Could you check a few things on this model? Use its own coordinates, in mm. A direction names the side the tool comes from. Round coordinates to 2 decimals unless told otherwise and drop trailing zeros. Write each loop counter-clockwise with the first axis right and the second up, starting at its lowest first coordinate (ties: lowest second). Pieces come first, ordered by that corner, then holes. Notation, with made-up numbers: M 23,-38 L 69,-38 A23 ccw 69,-19 Z; hole C 76.25,67 d9. An arc over 180 degrees is marked long. One line per item, written item: value. Start each with the question number.
(1) I'm going to push a flat-ended pin straight in: pin 1 Ø1 at (x, z) = (-28.5, 6.5) entering from +Y. Where does the tip first touch, or does it pass through?
(2) If I drill on L1, parallel to Z at x = 28, y = 0.5; L2, parallel to Z at x = 0, y = 3.05; L3, parallel to X at y = 0.4, z = -1.5, over which ranges is the centre line in solid material (lowest first)?
(3) I want a section at C-C on z = 0. Count the separate pieces of the cut face and the enclosed holes in it, and give its area (3 significant figures).
(4) Thinking about a two-plate mould opening in X: for faces 1 (the face through (49.638, 1.014, -0.189)), 2 (the face through (27, 2, -8.5)), 3 (the face through (-9, 2, 13.5)), which applies, released by +X, released by -X, zero draft, split by the parting line, or undercut?
(5) Which directions (+Z, -Z, +X, -X, +Y, -Y) give clear straight access to the entire face, cutting with the end or side of a thin tool? Please do faces 4 (the face through (1, 4, 6)), 5 (the face through (41.498, 1.972, -0.187)).
(6) I want a section at D-D on x = -30.5. Please give me the cut outline in (y, z).
(7) I want a section at B-B on y = 3.25. Please give me the cut outline in (x, z), and give its area (3 significant figures).
(8) I want a section at A-A on x = 0. Please give me the cut outline in (y, z), and give its area (3 significant figures).
Autodesk Inventor part; units mm, degrees
ref_plane "YZ Plane" through (0, 0, 0) normal (1, 0, 0) x (0, 1, 0)
ref_plane "XZ Plane" through (0, 0, 0) normal (0, 1, 0) x (-1, 0, 0)
ref_plane "XY Plane" through (0, 0, 0) normal (0, 0, 1) x (1, 0, 0)
sketch "Sketch1" plane through (0, 0, 0) normal (0, 1, 0) x (-1, 0, 0)
  circle A0 centre (0, 0) radius 13.5
  circle A1 centre (0, 0) radius 60
  line L0 (-58.4615, -13.5) -> (58.4615, -13.5)
  line L1 (58.4615, -13.5) -> (58.4615, 13.5)
  line L2 (58.4615, 13.5) -> (-58.4615, 13.5)
  line L3 (-58.4615, 13.5) -> (-58.4615, -13.5)
  line L4 (-58.4615, -13.5) -> (58.4615, 13.5) construction
  line L5 (58.4615, -13.5) -> (-58.4615, 13.5) construction
  line L6 (-20, 0) -> (-33, 0) construction
  line L7 (-20, 8.5) -> (-33, 8.5)
  line L8 (-33, -8.5) -> (-20, -8.5)
  arc A2 (-20, -8.5) -> (-20, 8.5) centre (-20, 0) ccw
  arc A3 (-33, 8.5) -> (-33, -8.5) centre (-33, 0) ccw
  line L9 (-58.4615, -13.5) -> (-42.8731, 13.5)
  line L10 (-58.4615, -13.5) -> (-27.2846, -13.5) construction
  line L11 (33, 0) -> (20, 0) construction
  line L12 (33, 8.5) -> (20, 8.5)
  line L13 (20, -8.5) -> (33, -8.5)
  arc A4 (33, -8.5) -> (33, 8.5) centre (33, 0) ccw
  arc A5 (20, 8.5) -> (20, -8.5) centre (20, 0) ccw
  line L14 (58.4615, 13.5) -> (47.2814, -5.8645)
  line L15 (58.4615, 13.5) -> (80.8217, 13.5) construction
  line L16 (47.2814, -5.8645) -> (42.8731, -13.5)
  point P0 (0, 0)
  point P1 (-0.767, 13.4782)
  point P2 (-9.0908, 9.9804)
  point P3 (0, 0)
  point P4 (-26.5, 0)
  point P5 (26.5, 0)
  point P6 (45.9853, -13.5)
  point P7 (0, 13.5)
  point P8 (0, -13.5)
  point P9 (12.75, -4.4371)
  point P10 (12.75, 4.4371)
  point P11 (-12.75, 4.4371)
  point P12 (-12.75, -4.4371)
  dimension "d7" = 120
  dimension "d1" = 27
  dimension "d9" = 5
  dimension "d10" = 5
  dimension "d11" = 60
  dimension "d12" = 5
  dimension "d13" = 5
  dimension "d14" = 13
  dimension "d15" = 13
  dimension "d16" = 20
  dimension "d17" = 20
  dimension "d24" = 120
extrude "Extrusion1" add sketch "Sketch1" along normal blind 4 contours A5 A0 A2 | A0 L2 L14 L16 L0 A5 L13 A4 L12 | A0 A2 L7 A3 L8 L0 L9 L2
chamfer "Chamfer1" distance 2 angle 45 4 edges at (50.6673, 4, 0) (50.6673, 0, 0) (-52.8715, 0, 3.8177) (-52.8715, 4, 3.8177)
sketch "Sketch2" plane through (0, 4, 0) normal (0, 1, 0) x (1, 0, 0)
  circle A0 centre (0, 0) radius 4
  line L0 (0, 0) -> (7.0711, -7.0711)
  line L1 (0, 0) -> (10, 0) construction
  circle A1 centre (7.0711, -7.0711) radius 1.5
  circle A2 centre (7.0711, 7.0711) radius 1.5
  circle A3 centre (-7.0711, 7.0711) radius 1.5
  circle A4 centre (-7.0711, -7.0711) radius 1.5
  dimension "d21" = 8
  dimension "d31" = 10
  dimension "d32" = 45
  dimension "d33" = 3
  dimension "d36" = 360
extrude "Extrusion2" cut sketch "Sketch2" against normal blind 4
equation "\"d10\" = d9"
equation "\"d12\" = d9"
equation "\"d13\" = d9"
equation "\"d15\" = d14"
properties part number "rotorV2"
Found:
1. pin 1: passes through
2. L1: z = -13.5 to -8.5, 8.5 to 13.5
2. L2: z = -13.5 to -4, 4 to 13.5
2. L3: x = -47.95 to -41.37, -11.63 to -3.71, 3.71 to 11.63, 41.37 to 49.69
3. separate pieces: 4
3. enclosed holes: 0
3. area: 124 mm²
4. face 1: released by +X
4. face 2: undercut
4. face 3: zero draft
5. face 4: +Z, -Z, +X, -X, +Y
5. face 5: +Y, -Y
6. outline: M 0,-13.5 L 4,-13.5 L 4,-8.5 L 0,-8.5 Z; M 0,8.5 L 4,8.5 L 4,13.5 L 0,13.5 Z
7. outline: M -57.02,13.5 L -46.2,-5.24 L -41.43,-13.5 L 57.02,-13.5 L 41.43,13.5 Z; hole M -33,-8.5 L -20,-8.5 A8.5 ccw -20,8.5 L -33,8.5 A8.5 ccw Z; hole C -7.07,-7.07 d3; hole C -7.07,7.07 d3; hole C 0,0 d8; hole C 7.07,-7.07 d3; hole C 7.07,7.07 d3; hole M 20,-8.5 L 33,-8.5 A8.5 ccw 33,8.5 L 20,8.5 A8.5 ccw Z
7. area: 1,680 mm²
8. outline: M 0,-13.5 L 4,-13.5 L 4,-4 L 0,-4 Z; M 0,4 L 4,4 L 4,13.5 L 0,13.5 Z
8. area: 76.0 mm²
